from build123d import *

# Parameters (mm, degrees)
SKETCH1_W           = 34
SKETCH1_H           = 23
SKETCH1_R           = 2.5
BOSS_EXTRUDE1_DEPTH = 23
SKETCH6_OUTSIDE_W   = 45.41
SKETCH6_OUTSIDE_H   = 34.41
SKETCH6_OUTSIDE_W_2 = 34
SKETCH6_OUTSIDE_H_2 = 23
SKETCH6_OUTSIDE_R   = 2.5
CUT_EXTRUDE10_DEPTH = 24
SKETCH7_OUTSIDE_W   = 34.41
SKETCH7_OUTSIDE_H   = 34.41
SKETCH7_OUTSIDE_W_2 = 23
SKETCH7_OUTSIDE_H_2 = 23
SKETCH7_OUTSIDE_W_3 = 17.08
SKETCH7_OUTSIDE_H_3 = 17.08
CUT_EXTRUDE11_DEPTH = 34
BOSS_EXTRUDE2_DEPTH = 23
SKETCH13_R          = 2.5
BOSS_EXTRUDE3_DEPTH = 4


with BuildPart() as part:
    # sketch1 → Boss-Extrude1 (new body)
    with BuildSketch(Plane(origin=(0, 0, 0), x_dir=(1, 0, 0), z_dir=(0, 1, 0))):
        with Locations((17, -11.5)):
            Rectangle(SKETCH1_W, SKETCH1_H)
        with Locations((8.5, -11.5)):
            Circle(SKETCH1_R, mode=Mode.SUBTRACT)
        with Locations((25.5, -11.5)):
            Circle(SKETCH1_R, mode=Mode.SUBTRACT)
    extrude(amount=BOSS_EXTRUDE1_DEPTH)

    # Sketch6 outside → Cut-Extrude10 (cut, through all)
    with BuildSketch(Plane(origin=(0, 0, 0), x_dir=(-1, 0, 0), z_dir=(0, 0, -1))):
        with Locations((-17, 11.5)):
            Rectangle(SKETCH6_OUTSIDE_W, SKETCH6_OUTSIDE_H)
        with Locations((-17, 11.5)):
            Rectangle(SKETCH6_OUTSIDE_W_2, SKETCH6_OUTSIDE_H_2, mode=Mode.SUBTRACT)
        with Locations((-25.5, 11.5)):
            Circle(SKETCH6_OUTSIDE_R)
        with Locations((-8.5, 11.5)):
            Circle(SKETCH6_OUTSIDE_R)
    extrude(amount=-CUT_EXTRUDE10_DEPTH, mode=Mode.SUBTRACT)

    # Sketch7 outside → Cut-Extrude11 (cut)
    with BuildSketch(Plane(origin=(34, 0, 0), x_dir=(0, 0, -1), z_dir=(1, 0, 0))):
        with Locations((-11.5, 11.5)):
            Rectangle(SKETCH7_OUTSIDE_W, SKETCH7_OUTSIDE_H)
        with Locations((-11.5, 11.5)):
            Rectangle(SKETCH7_OUTSIDE_W_2, SKETCH7_OUTSIDE_H_2, mode=Mode.SUBTRACT)
        with Locations((-11.5, 11.5)):
            Rectangle(SKETCH7_OUTSIDE_W_3, SKETCH7_OUTSIDE_H_3)
    extrude(amount=-CUT_EXTRUDE11_DEPTH, mode=Mode.SUBTRACT)


with BuildPart() as body_2:
    # Mirror6: mirrored copy
    add(part.part.mirror(Plane(origin=(0, 0, 0), x_dir=(-0.707106781, 0, 0.707106781), z_dir=(-0.707106781, 0, -0.707106781))))


with BuildPart() as part_1:
    add(part.part)

    add(body_2.part)  # Boss-Extrude2 merges body 2
    # Sketch11 → Boss-Extrude2 (add)
    with BuildSketch(Plane(origin=(0, 0, 0), x_dir=(1, 0, 0), z_dir=(0, 1, 0))):
        Polygon((-23, 0), (0, -23), (0, 0), align=None)
    extrude(amount=BOSS_EXTRUDE2_DEPTH)

    # Sketch13 → Boss-Extrude3 (add)
    with BuildSketch(Plane(origin=(0, 0, 0), x_dir=(1, 0, 0), z_dir=(0, 1, 0))):
        Polygon((8.706365938, 8.706365938), (0, 17), (0, 0), (17, 0), align=None)
        with Locations((5.170832032, 5.170832032)):
            Circle(SKETCH13_R, mode=Mode.SUBTRACT)
    extrude(amount=BOSS_EXTRUDE3_DEPTH)


solid = part_1.part
Can you work these out from the model? Positions are in its coordinate system, mm. A direction names the side the tool comes from. Give positions to 0.01 mm unless a question says otherwise; leave off trailing zeros. Order: outer loops, then holes, each group sorted by start corner. A loop starts at its lowest first (then second) coordinate and runs counter-clockwise, first axis right, second up. Notation, with made-up numbers: M 20,85 L 79,85 A17 cw 79,115 Z; hole C -1,16.5 d6. An arc over 180 degrees is marked long. One line per item, written item: value.
Item 1: For faces 4 (the face through (6, 4, -9)), 5 (the face through (17, 2.96, 12)), 6 (the face through (-1, 0, 0)), 7 (the face through (-12, 20.04, -17)), which set-ups out of +Z, -Z, +X, -X, +Y, -Y let a thin tool reach every point of the face, with its end or its side?
Verdict:
face 4: -Z, +X, +Y
face 5: +X
face 6: +Z, -Z, +X, -X, -Y
face 7: -Z
Item 2: If we section it at C-C on x = 5: Write out the boundary of the cut face in (y, z).
Verdict:
outline: M 0,-12.24 L 4,-12.24 L 4,-7.66 L 0,-7.66 Z; M 0,-2.68 L 4,-2.68 L 4,0 L 23,0 L 23,23 L 0,23 Z; hole M 2.96,2.96 L 20.04,2.96 L 20.04,20.04 L 2.96,20.04 Z
Item 3: If we section it at D-D on y = 6.5: Write out the boundary of the cut face in (x, z), and give its area (3 significant figures).
Verdict:
outline: M -23,-34 L -20.04,-34 L -20.04,0 L -2.96,0 L -2.96,-34 L 0,-34 L 0,0 L 34,0 L 34,2.96 L 0,2.96 L 0,20.04 L 34,20.04 L 34,23 L 0,23 L -23,0 Z
area: 667 mm2
Item 4: If we section it at B-B on z = -30: Write out the boundary of the cut face in (x, y), and give its area (3 significant figures).
Verdict:
outline: M -23,0 L 0,0 L 0,23 L -23,23 Z; hole M -20.04,2.96 L -2.96,2.96 L -2.96,20.04 L -20.04,20.04 Z
area: 237 mm2
Item 5: For pin 1 (12 mm diameter, centred on y = 4.5, z = -20.5, fed in from +X); pin 2 (2 mm diameter, centred on x = -1.5, y = 15.5, fed in from +Z); pin 3 (6 mm diameter, centred on x = 8.5, y = 11.5, fed in from +Z); pin 4 (8.5 mm diameter, centred on x = 17.5, y = 14, fed in from -Z), each with a flat end and sliding along its axis, tell me the tip position at first contact or that it passes through.
Verdict:
pin 1: x = 2.6
pin 2: z = 22.5
pin 3: z = 23
pin 4: z = 0
Item 6: If we section it at A-A on x = 25.5: Write out the boundary of the cut face in (y, z), and give its area (3 significant figures).
Verdict:
outline: M 0,0 L 9,0 L 9,2.96 L 2.96,2.96 L 2.96,9 L 0,9 Z; M 0,14 L 2.96,14 L 2.96,20.04 L 9,20.04 L 9,23 L 0,23 Z; M 14,0 L 23,0 L 23,9 L 20.04,9 L 20.04,2.96 L 14,2.96 Z; M 14,20.04 L 20.04,20.04 L 20.04,14 L 23,14 L 23,23 L 14,23 Z
area: 178 mm2
Item 7: If we mould it in two halves opening along X, with no side actions, what happens to faces 1 (the face through (24.96, 21.5, 13.94)), 2 (the face through (0, 14, -17)), 3 (the face through (-21.5, 10, -27.5))? For each: pulls with the +X half, pulls with the -X half, needs draft (parallel to the pull), parting line crosses it, or undercut.
Verdict:
face 1: undercut
face 2: pulls with the +X half
face 3: needs draft
Item 8: Please list where these lines run through material, in increasing order: line 1 (Y direction, x = -7, z = -6); line 2 (X direction, y = 6.5, z = -8).
Verdict:
line 1: 0 to 2.96, 20.04 to 23
line 2: -23 to -20.04, -2.96 to 0
